Work out the finished part from the listing and answer in its coordinate system (mm). A direction names the side the tool comes from. Give positions to 0.01 mm unless a question says otherwise; leave off trailing zeros. Order: outer loops, then holes, each group sorted by start corner. A loop starts at its lowest first (then second) coordinate and runs counter-clockwise, first axis right, second up.
```python
from build123d import *

# Parameters (mm, degrees)
SKETCH1_W           = 10.8
SKETCH1_H           = 25.2
BOSS_EXTRUDE1_DEPTH = 10.55
SKETCH2_R           = 4.565
BOSS_EXTRUDE2_DEPTH = 7.7
SKETCH3_R           = 4.565
BOSS_EXTRUDE3_DEPTH = 7.7
SKETCH4_W           = 2
SKETCH4_H           = 0.8
SKETCH5_W           = 2
SKETCH5_H           = 0.8
BOSS_EXTRUDE4_DEPTH = 4.6
SKETCH7_W           = 7.17
SKETCH7_H           = 12.01
CUT_EXTRUDE1_DEPTH  = 3.6
SKETCH8_W           = 3.73
SKETCH8_H           = 10.95
BOSS_EXTRUDE5_DEPTH = 9.38
SKETCH9_R           = 1.8
BOSS_EXTRUDE6_DEPTH = 10
SKETCH11_R          = 1.825
BOSS_EXTRUDE7_DEPTH = 10


with BuildPart() as part:
    # Sketch1 → Boss-Extrude1 (new body)
    with BuildSketch(Plane(origin=(0, 0, 0), x_dir=(1, 0, 0), z_dir=(0, 1, 0))):
        Rectangle(SKETCH1_W, SKETCH1_H)
    extrude(amount=BOSS_EXTRUDE1_DEPTH)

    # Sketch2 → Boss-Extrude2 (add)
    with BuildSketch(Plane.XY.offset(12.6)):
        with Locations((0, 5.403958649)):
            Circle(SKETCH2_R)
    extrude(amount=BOSS_EXTRUDE2_DEPTH)

    # Sketch3 → Boss-Extrude3 (add)
    with BuildSketch(Plane(origin=(0, 0, -12.6), x_dir=(-1, 0, 0), z_dir=(0, 0, -1))):
        with Locations((0, 5.344439272)):
            Circle(SKETCH3_R)
    extrude(amount=BOSS_EXTRUDE3_DEPTH)

    # Sketch4 → Cut-Revolve1 (revolve, cut)
    with BuildSketch(Plane(origin=(0, 0, 0), x_dir=(0, 0, -1), z_dir=(1, 0, 0))):
        with Locations((-17.43, 9.568958649)):
            Rectangle(SKETCH4_W, SKETCH4_H)
    revolve(axis=Axis((0, 5.403958649, 20.3), (0, 0, -1)), mode=Mode.SUBTRACT)

    # Sketch5 → Cut-Revolve2 (revolve, cut)
    with BuildSketch(Plane(origin=(0, 0, 0), x_dir=(0, 0, -1), z_dir=(1, 0, 0))):
        with Locations((17.43, 9.509439272)):
            Rectangle(SKETCH5_W, SKETCH5_H)
    revolve(axis=Axis((0, 5.344439272, -20.3), (0, 0, 1)), mode=Mode.SUBTRACT)

    # Sketch6 → Boss-Extrude4 (add)
    with BuildSketch(Plane(origin=(0, 10.55, 0), x_dir=(1, 0, 0), z_dir=(0, 1, 0))):
        with BuildLine():
            Line((4.595, -5.465), (4.595, 5.465))
            ThreePointArc((4.595, 5.465), (0, 10.06), (-4.595, 5.465))
            Line((-4.595, 5.465), (-4.595, -5.465))
            ThreePointArc((-4.595, -5.465), (0, -10.06), (4.595, -5.465))
        make_face()
    extrude(amount=BOSS_EXTRUDE4_DEPTH)

    # Sketch7 → Cut-Extrude1 (cut)
    with BuildSketch(Plane(origin=(0, 15.15, 0), x_dir=(1, 0, 0), z_dir=(0, 1, 0))):
        Rectangle(SKETCH7_W, SKETCH7_H)
    extrude(amount=-CUT_EXTRUDE1_DEPTH, mode=Mode.SUBTRACT)

    # Sketch8 → Boss-Extrude5 (add)
    with BuildSketch(Plane(origin=(0, 11.55, 0), x_dir=(1, 0, 0), z_dir=(0, 1, 0))):
        Rectangle(SKETCH8_W, SKETCH8_H)
    extrude(amount=BOSS_EXTRUDE5_DEPTH)

    # Sketch9 → Boss-Extrude6 (add)
    with BuildSketch(Plane(origin=(0, 0, -20.3), x_dir=(-1, 0, 0), z_dir=(0, 0, -1))):
        with Locations((0, 5.407254025)):
            Circle(SKETCH9_R)
    extrude(amount=BOSS_EXTRUDE6_DEPTH)

    # Sketch11 → Boss-Extrude7 (add)
    with BuildSketch(Plane.XY.offset(20.3)):
        with Locations((0, 5.564693588)):
            Circle(SKETCH11_R)
    extrude(amount=BOSS_EXTRUDE7_DEPTH)


solid = part.part
```
1. The part is cut by section D-D (z = -17.5). Write down the section's boundary in (x, y) (3 decimals), then the cut area to 3 significant figures.
Findings below:
outline: circle Ø7.53 at (0, 5.344)
area: 44.5 mm2
2. The part is cut by section B-B (y = 18.25). Write down the section's boundary in (x, z) (3 decimals), then the cut area to 3 significant figures.
Findings below:
outline: (-1.865, -5.475) - (1.865, -5.475) - (1.865, 5.475) - (-1.865, 5.475) - close
area: 40.8 mm2
3. The part is cut by section A-A (z = 2). Write down the section's boundary in (x, y) (3 decimals), then the cut area to 3 significant figures.
Findings below:
outline: (-5.4, 0) - (5.4, 0) - (5.4, 10.55) - (4.595, 10.55) - (4.595, 15.15) - (3.585, 15.15) - (3.585, 11.55) - (1.865, 11.55) - (1.865, 20.93) - (-1.865, 20.93) - (-1.865, 11.55) - (-3.585, 11.55) - (-3.585, 15.15) - (-4.595, 15.15) - (-4.595, 10.55) - (-5.4, 10.55) - close
area: 165 mm2
4. The part is cut by section C-C (y = 2.25). Write down the section's boundary in (x, z).
Findings below:
outline: (-5.4, -12.6) - (-3.36, -12.6) - (-3.36, -16.43) - (-2.14, -16.43) - (-2.14, -18.43) - (-3.36, -18.43) - (-3.36, -20.3) - (3.36, -20.3) - (3.36, -18.43) - (2.14, -18.43) - (2.14, -16.43) - (3.36, -16.43) - (3.36, -12.6) - (5.4, -12.6) - (5.4, 12.6) - (3.3, 12.6) - (3.3, 16.43) - (2.06, 16.43) - (2.06, 18.43) - (3.3, 18.43) - (3.3, 20.3) - (-3.3, 20.3) - (-3.3, 18.43) - (-2.06, 18.43) - (-2.06, 16.43) - (-3.3, 16.43) - (-3.3, 12.6) - (-5.4, 12.6) - close
5. Which of the six approach directions +Z, -Z, +X, -X, +Y, -Y give full straight-line access (tool end or side, diameter ignored) to faces 4 (the face through (4.354, 6.775, 14.488)), 5 (the face through (-0.1, 12.82, 10.06)), 6 (the face through (3.585, 13, 0))?
Findings below:
face 4: +Z
face 5: +Z, +Y
face 6: +Y
6. Given P1, Ø4.5, axis at y = 14.5, z = 2.5, coming from the -X side (3 decimals); P2, Ø1, axis at y = 5.5, z = -18, coming from the +X side (3 decimals); P3, Ø4, axis at x = -0.5, y = 16.5, coming from the -Z side, each flat-ended and moving along its own axis, determine where each tip first touches the part or whether it passes through.
Findings below:
P1: stops at x = -4.595
P2: stops at x = 4.565
P3: stops at z = -10.06
7. Straight lines are drawn through the part: probe 1 along Z at (x, y) = (-2.5, 2); probe 2 along Z at (x, y) = (-4.5, 9); probe 3 along Y at (x, z) = (-2.5, -7). For each, find the intervals that lie inside material, in ascending order.
Findings below:
probe 1: z = -20.3 to -18.43, -16.43 to 16.43, 18.43 to 20.3
probe 2: z = -12.6 to 12.6
probe 3: y = 0 to 15.15
8. The mould has two halves that part along X. Classify faces 1 (the face through (4, 15.15, 0)), 2 (the face through (0.234, 7.192, -25.23)), 3 (the face through (0, 16, -5.475)): pulls with the +X half, pulls with the -X half, needs draft (parallel to the pull), parting line crosses it, or undercut.
Findings below:
face 1: needs draft
face 2: parting line crosses it
face 3: undercut
